```python
from build123d import *

# Parameters (mm, degrees)
SKETCH1_W           = 63.6
SKETCH1_H           = 39.1
BOSS_EXTRUDE1_DEPTH = 23
SKETCH3_W           = 47.08
SKETCH3_H           = 23.12
BOSS_EXTRUDE2_DEPTH = 4.6
SKETCH4_W           = 29.3
SKETCH4_H           = 16.4
BOSS_EXTRUDE3_DEPTH = 10.9
SHELL1_T            = -3
SKETCH5_W           = 123.6
SKETCH5_H           = 39.1
BOSS_EXTRUDE4_DEPTH = 3
SKETCH6_R           = 1.73
CUT_EXTRUDE1_DEPTH  = 110.599361312
SKETCH7_W           = 57.6
SKETCH7_H           = 33.1
CUT_EXTRUDE2_DEPTH  = 3
SKETCH8_R           = 1.8
CUT_EXTRUDE3_DEPTH  = 3
FILLET1_R           = 10
SKETCH9_R           = 5.15
CUT_EXTRUDE4_DEPTH  = 10
SKETCH12_R          = 5.15
CUT_EXTRUDE5_DEPTH  = 110.599361312


with BuildPart() as part:
    # Sketch1 → Boss-Extrude1 (new body)
    with BuildSketch(Plane(origin=(0, 0, 0), x_dir=(1, 0, 0), z_dir=(0, 1, 0))):
        with Locations((31.8, 19.55)):
            Rectangle(SKETCH1_W, SKETCH1_H)
    extrude(amount=BOSS_EXTRUDE1_DEPTH)

    # Sketch3 → Boss-Extrude2 (add)
    with BuildSketch(Plane(origin=(0, 23, 0), x_dir=(1, 0, 0), z_dir=(0, 1, 0))):
        with Locations((32.62, 19.55)):
            Rectangle(SKETCH3_W, SKETCH3_H)
    extrude(amount=BOSS_EXTRUDE2_DEPTH)

    # Sketch4 → Boss-Extrude3 (add)
    with BuildSketch(Plane(origin=(0, 27.6, 0), x_dir=(1, 0, 0), z_dir=(0, 1, 0))):
        with Locations((25.45, 19.55)):
            Rectangle(SKETCH4_W, SKETCH4_H)
    extrude(amount=BOSS_EXTRUDE3_DEPTH)

    # Shell1
    shell1_openings = [part.faces().sort_by_distance(p)[0] for p in [
        (31.8, 0, -19.55),
    ]]
    offset(amount=SHELL1_T, openings=shell1_openings, kind=Kind.INTERSECTION)

    # Sketch5 → Boss-Extrude4 (add)
    with BuildSketch(Plane.XZ):
        with Locations((31.8, -19.55)):
            Rectangle(SKETCH5_W, SKETCH5_H)
    extrude(amount=BOSS_EXTRUDE4_DEPTH)

    # Sketch6 → Cut-Extrude1 (cut, through all)
    with BuildSketch(Plane(origin=(0, 38.5, 0), x_dir=(1, 0, 0), z_dir=(0, 1, 0))):
        with Locations(Location((18.95, 19.55, 0), (0, 0, 270))):
            Circle(SKETCH6_R)
        with Locations(Location((31.65, 19.55, 0), (0, 0, 270))):
            Circle(SKETCH6_R)
    extrude(amount=-CUT_EXTRUDE1_DEPTH, mode=Mode.SUBTRACT)

    # Sketch7 → Cut-Extrude2 (cut)
    with BuildSketch(Plane.XZ.offset(3)):
        with Locations((31.8, -19.55)):
            Rectangle(SKETCH7_W, SKETCH7_H)
    extrude(amount=-CUT_EXTRUDE2_DEPTH, mode=Mode.SUBTRACT)

    # Sketch8 → Cut-Extrude3 (cut)
    with BuildSketch(Plane(origin=(0, 0, 0), x_dir=(1, 0, 0), z_dir=(0, 1, 0))):
        with Locations(Location((85.6, 8, 0), (0, 0, 270))):
            Circle(SKETCH8_R)
        with Locations(Location((71.6, 31.1, 0), (0, 0, 270))):
            Circle(SKETCH8_R)
        with Locations(Location((-8, 8, 0), (0, 0, 270))):
            Circle(SKETCH8_R)
        with Locations(Location((-22, 31.1, 0), (0, 0, 270))):
            Circle(SKETCH8_R)
    extrude(amount=-CUT_EXTRUDE3_DEPTH, mode=Mode.SUBTRACT)

    # Fillet1
    fillet1_edges = [part.edges().sort_by_distance(p)[0] for p in [
        (93.6, -1.5, -39.1),
        (93.6, -1.5, 0),
        (-30, -1.5, 0),
        (-30, -1.5, -39.1),
    ]]
    fillet(fillet1_edges, radius=FILLET1_R)

    # Sketch9 → Cut-Extrude4 (cut)
    with BuildSketch(Plane(origin=(0, 27.6, 0), x_dir=(1, 0, 0), z_dir=(0, 1, 0))):
        with Locations(Location((44.35, 19.55, 0), (0, 0, 214.386893027))):
            Circle(SKETCH9_R)
    extrude(amount=-CUT_EXTRUDE4_DEPTH, mode=Mode.SUBTRACT)

    # Sketch12 → Cut-Extrude5 (cut, through all)
    with BuildSketch(Plane(origin=(0, 38.5, 0), x_dir=(1, 0, 0), z_dir=(0, 1, 0))):
        with Locations(Location((44.35, 19.55, 0), (0, 0, 214.386893027))):
            Circle(SKETCH12_R)
    extrude(amount=-CUT_EXTRUDE5_DEPTH, mode=Mode.SUBTRACT)


solid = part.part
```
Build history of the part. All positions in model axes, mm. A direction names the side the tool comes from. Coordinates: 2 decimals unless noted, no trailing zeros. Order: outer loops, then holes, each group sorted by start corner. A loop starts at its lowest first (then second) coordinate and runs counter-clockwise, first axis right, second up. Notation, with made-up numbers: M -5,29.25 L 39,29.25 A16 ccw 39,45.25 Z; hole C 51.25,80.5 d6. An arc over 180 degrees is marked long. One line per question, with ' | ' between items. Start each with the question number.
1. Tool access for faces 1 (the face through (9.08, 25, -19)), 2 (the face through (78, 0, -19)), 3 (the face through (60.6, 8, -20)): list every direction of +Z, -Z, +X, -X, +Y, -Y with a clear straight run to the whole face (end or side of a thin tool).
2. Wall check: line 1 along Z through (x, y) = (6.5, 13); line 2 along X through (y, z) = (-1.3, -31.1); line 3 along X through (y, z) = (1, -20.5). Give the ranges that are in metal, low to high. Write a range as [from, to].
3. Flat gauge pins, fed straight in: P1, Ø5.5, axis at x = 24, y = 31, coming from the -Z side; P2, Ø8.5, axis at x = 29, z = -17, coming from the -Y side; P3, Ø5, axis at y = 24.5, z = -24.5, coming from the +X side. Where does each tip first touch, or does it go through?
4. Cut at A-A (x = -8). Write the cut outline in (y, z).
5. Cut at D-D (x = 23). Write the cut outline in (y, z), plus the area to 3 significant figures.
6. Mould opens along Z. For faces 4 (the face through (32, 22, -28.11)), 5 (the face through (25, 33, -11.35)), 6 (the face through (-15, 0, -19)) say: +Z half, -Z half, draft (parallel to the pull), parting line (faces both ways), or undercut.
7. Cut at B-B (y = 26). Write the cut outline in (x, z).
8. Cut at C-C (y = 5). Write the cut outline in (x, z).
The answers:
1) face 1: +Z, -Z, -X, +Y | face 2: +Z, -Z, +X, +Y | face 3: -Y
2) line 1: z = [-39.1, -36.1], [-3, 0] | line 2: x = [-29.8, -23.8], [-20.2, 3], [60.6, 69.8], [73.4, 93.4] | line 3: x = [0, 3], [60.6, 63.6]
3) P1: stops at z = -27.75 | P2: stops at y = 24.6 | P3: stops at x = 63.6
4) outline: M -3,-39.1 L 0,-39.1 L 0,-9.8 L -3,-9.8 Z; M -3,-6.2 L 0,-6.2 L 0,0 L -3,0 Z
5) outline: M -3,-39.1 L 23,-39.1 L 23,-31.11 L 27.6,-31.11 L 27.6,-27.75 L 38.5,-27.75 L 38.5,-11.35 L 27.6,-11.35 L 27.6,-7.99 L 23,-7.99 L 23,0 L -3,0 L -3,-3 L 20,-3 L 20,-10.99 L 24.6,-10.99 L 24.6,-14.35 L 35.5,-14.35 L 35.5,-24.75 L 24.6,-24.75 L 24.6,-28.11 L 20,-28.11 L 20,-36.1 L -3,-36.1 Z | area: 348 mm2
6) face 4: undercut | face 5: +Z half | face 6: draft
7) outline: M 9.08,-31.11 L 56.16,-31.11 L 56.16,-7.99 L 9.08,-7.99 Z; hole M 13.8,-24.75 L 37.1,-24.75 L 37.1,-14.35 L 13.8,-14.35 Z; hole C 44.35,-19.55 d10.3
8) outline: M 0,-39.1 L 63.6,-39.1 L 63.6,0 L 0,0 Z; hole M 3,-36.1 L 60.6,-36.1 L 60.6,-3 L 3,-3 Z
